Model file for the job. Use its own axes, mm. Round coordinates to 2 decimals unless told otherwise and drop trailing zeros. Order: outer loops, then holes, each group sorted by start corner. A loop starts at its lowest first (then second) coordinate and runs counter-clockwise, first axis right, second up. Notation, with made-up numbers: (43.5, 1) - (51.5, 1) arc R20 cw to (51.5, 17) - close; hole circle Ø11 at (18, -39). An arc over 180 degrees is marked (long way). Write item = value, one per line. Start each with the question number.
Autodesk Inventor part; units mm, degrees
ref_plane "YZ Plane" through (0, 0, 0) normal (1, 0, 0) x (0, 1, 0)
ref_plane "XZ Plane" through (0, 0, 0) normal (0, 1, 0) x (-1, 0, 0)
ref_plane "XY Plane" through (0, 0, 0) normal (0, 0, 1) x (1, 0, 0)
sketch "Boceto1" plane through (0, 0, 0) normal (0, 1, 0) x (-1, 0, 0)
  line L0 (20, 30) -> (-76, 30)
  line L1 (-76, 30) -> (-76, -30)
  line L2 (-76, -30) -> (20, -30)
  line L3 (20, -30) -> (20, 30)
  line L4 (-3, -25) -> (-58, -25) construction
  line L5 (-58, -25) -> (-58, 15) construction
  line L6 (-58, 15) -> (-3, 15) construction
  line L7 (-3, 15) -> (-3, -25) construction
  circle A0 centre (-58, -25) radius 1.5
  circle A1 centre (-3, -25) radius 1.5
  circle A2 centre (-3, 15) radius 1.5
  circle A3 centre (-58, 15) radius 1.5
  point P0 (0, 0)
  point P1 (20, 0)
  dimension "d0" = 3
  dimension "d1" = 60
  dimension "d2" = 18
  dimension "d5" = 96
  dimension "d6" = 20
  dimension "d7" = 15
  dimension "d8" = 5
  dimension "d9" = 55
extrude "Extrusión1" add sketch "Boceto1" against normal blind 2.5
properties part number "placa circuito"
Item 1: Saw through at B-B, the plane z = -25. Give the cut face in (x, y).
Item 2: Probe L1, parallel to Z at x = 3, y = -0.7; L2, parallel to X at y = -2.25, z = -24. List the from-to ranges inside material, lowest first.
Item 3: Saw through at A-A, the plane x = 58. Give the cut face in (y, z), then the cut area to 3 significant figures.
Item 4: Mould opens along Z. For faces 1 (the face through (3.195, -1.232, -23.513)), 2 (the face through (29, -2.5, 0)), 3 (the face through (29, -1, -30)) say: +Z half, -Z half, draft (parallel to the pull), parting line (faces both ways), or undercut.
Check sheet entries:
q1.outline = (-20, -2.5) - (1.5, -2.5) - (1.5, 0) - (-20, 0) - close; (4.5, -2.5) - (56.5, -2.5) - (56.5, 0) - (4.5, 0) - close; (59.5, -2.5) - (76, -2.5) - (76, 0) - (59.5, 0) - close
q2.L1 = -30 to -26.5, -23.5 to 13.5, 16.5 to 30
q2.L2 = -20 to 1.88, 4.12 to 56.88, 59.12 to 76
q3.outline = (-2.5, -30) - (0, -30) - (0, -26.5) - (-2.5, -26.5) - close; (-2.5, -23.5) - (0, -23.5) - (0, 13.5) - (-2.5, 13.5) - close; (-2.5, 16.5) - (0, 16.5) - (0, 30) - (-2.5, 30) - close
q3.area = 135 mm2
q4.face_1 = undercut
q4.face_2 = draft
q4.face_3 = -Z half
